Here's how the part is built. I have some questions about the finished solid (model axes, mm). Face numbers are marked on the shaded views. A direction names the side the tool comes from. Coordinates: 2 decimals unless noted, no trailing zeros. Write each loop counter-clockwise with the first axis right and the second up, starting at its lowest first coordinate (ties: lowest second). Pieces come first, ordered by that corner, then holes. Notation, with made-up numbers: M 25.25,88 L 59.25,88 A23 ccw 59.25,102 Z; hole C 29.5,41.5 d5. An arc over 180 degrees is marked long. Use one line per item in the form item = value. Start each with the question number.
1. Please list where these lines run through material, in increasing order: line 1 along Z through (x, y) = (30, -7.75); line 2 along X through (y, z) = (-1.25, -7); line 3 along Z through (x, y) = (28.5, -3.25). Write a range as [from, to].
2. I want a section at B-B, the plane y = -2.5. Count the separate pieces of the cut face and the enclosed holes in it, plus the area to 3 significant figures.
3. I'm going to push flat-ended pins straight in: pin 1 Ø5 at (x, y) = (33.5, -3) entering from +Z; pin 2 Ø11 at (y, z) = (-7, -0.5) entering from -X; pin 3 Ø1.5 at (x, z) = (-10.5, -3) entering from -Y. Where does each tip first touch, or does it pass through?
4. I want a section at C-C, the plane x = 3. List the corners of the cut face in (y, z) for me, plus the area to 3 significant figures.
5. I want a section at A-A, the plane z = 12. List the corners of the cut face in (x, y) for me, plus the area to 3 significant figures.
6. On a 3-axis mill with a long thin cutter (end or side, diameter ignored), from which of +Z, -Z, +X, -X, +Y, -Y can I reach the whole of each face in a straight line? I mean the marked faces 5, 6, 7, 8 and 9. Say none if no direction works.
7. Thinking about a two-plate mould opening in X: for the marked faces 1, 2, 3 and 4, which applies, released by +X, released by -X, zero draft, split by the parting line, or undercut?
from build123d import *
from build123d.topology import SkipClean

# Parameters (mm, degrees)
EXTRUDE_1_DEPTH       = 20
EXTRUDE_1_DEPTH_BACK  = 20
EXTRUDE_2_DEPTH       = 15
EXTRUDE_2_DEPTH_BACK  = 15
HOLE_WIZARD_M51_D     = 4.2
HOLE_WIZARD_M51_DEPTH = 16
HOLE_WIZARD_M51_TIP   = 1.2618073
CHAMFER_1_SIZE        = 3
FILLET_1_R            = 0.2
FILLET_2_R            = 0.2
FILLET_3_R            = 0.2


with BuildPart() as part:
    # Эскиз1 → Бобышка-Вытянуть1 (new, two sides: drawn at the far end of the back side and taken through both)
    with BuildSketch(Plane.XY.offset(-EXTRUDE_1_DEPTH_BACK)):
        with BuildLine():
            Line((17.5, -12.5), (7.5, -12.5))
            Line((7.5, -12.5), (7.5, -20))
            Line((7.5, -20), (-7.5, -20))
            Line((-7.5, -20), (-7.5, -12.5))
            Line((-7.5, -12.5), (-17.5, -12.5))
            ThreePointArc((-17.5, -12.5), (-26.338834765, -8.838834765), (-30, 0))
            Line((-30, 0), (-25, 0))
            ThreePointArc((-25, 0), (-17.5, -7.5), (-10, 0))
            Line((-10, 0), (10, 0))
            ThreePointArc((10, 0), (17.5, -7.5), (25, 0))
            Line((25, 0), (30, 0))
            ThreePointArc((30, 0), (26.338834765, -8.838834765), (17.5, -12.5))
        make_face()
    extrude(amount=EXTRUDE_1_DEPTH + EXTRUDE_1_DEPTH_BACK)

    # Эскиз2 → Бобышка-Вытянуть2 (add, two sides: drawn at the far end of the back side and taken through both)
    with SkipClean():  # the faces are left unmerged after this step: merging them gives an invalid solid
        with BuildSketch(Plane.XY.offset(-EXTRUDE_2_DEPTH_BACK)):
            with BuildLine():
                Line((22.5, -25), (45, -25))
                Line((45, -25), (45, -10))
                Line((45, -10), (35, -10))
                Line((35, -10), (35, 0))
                Line((35, 0), (25, 0))
                ThreePointArc((25, 0), (17.5, -7.5), (10, 0))
                Line((10, 0), (-10, 0))
                ThreePointArc((-10, 0), (-17.5, -7.5), (-25, 0))
                Line((-25, 0), (-35, 0))
                Line((-35, 0), (-35, -10))
                Line((-35, -10), (-45, -10))
                Line((-45, -10), (-45, -25))
                Line((-45, -25), (-22.5, -25))
                Line((-22.5, -25), (-27.5, -20))
                Line((-27.5, -20), (27.5, -20))
                Line((27.5, -20), (22.5, -25))
            make_face()
        extrude(amount=EXTRUDE_2_DEPTH + EXTRUDE_2_DEPTH_BACK)
    add(part.part.scale(1), mode=Mode.REPLACE)  # the faces are merged on a copy

    # Отверстие обработанное метчиком M51
    with Locations(Plane(origin=(0, 0, 0), x_dir=(1, 0, 0), z_dir=(0, 1, 0))):
        with Locations((-30, 7.5), (-30, -7.5), (0, 15), (0, -15), (30, -7.5), (30, 7.5)):
            Hole(HOLE_WIZARD_M51_D / 2, depth=HOLE_WIZARD_M51_DEPTH)
            with Locations((0, 0, -(HOLE_WIZARD_M51_DEPTH + HOLE_WIZARD_M51_TIP / 2))):  # 118° drill point
                Cone(0, HOLE_WIZARD_M51_D / 2, HOLE_WIZARD_M51_TIP, mode=Mode.SUBTRACT)

    # Фаска1
    chamfer_1_edges = [part.edges().sort_by_distance(p)[0] for p in [
        (-45, -10, 0),
        (45, -10, 0),
    ]]
    chamfer(chamfer_1_edges, length=CHAMFER_1_SIZE)

    # Скругление1
    fillet_1_edges = [part.edges().sort_by_distance(p)[0] for p in [
        (27.5, -20, 0),
        (22.5, -25, 0),
        (-27.5, -20, 0),
        (-22.5, -25, 0),
    ]]
    fillet(fillet_1_edges, radius=FILLET_1_R)

    # Скругление2
    fillet_2_edges = [part.edges().sort_by_distance(p)[0] for p in [
        (-35, -10, 0),
    ]]
    fillet(fillet_2_edges, radius=FILLET_2_R)

    # Скругление3
    fillet_3_edges = [part.edges().sort_by_distance(p)[0] for p in [
        (-12.5, -12.5, 15),
        (-12.5, -12.5, -15),
        (12.5, -12.5, -15),
        (26.338834765, -8.838834765, -15),
        (7.5, -16.25, -15),
        (12.5, -12.5, 15),
        (26.338834765, -8.838834765, 15),
        (-26.338834765, -8.838834765, 15),
        (-7.5, -16.25, 15),
        (7.5, -16.25, 15),
        (-26.338834765, -8.838834765, -15),
        (-7.5, -16.25, -15),
    ]]
    fillet(fillet_3_edges, radius=FILLET_3_R)


solid = part.part
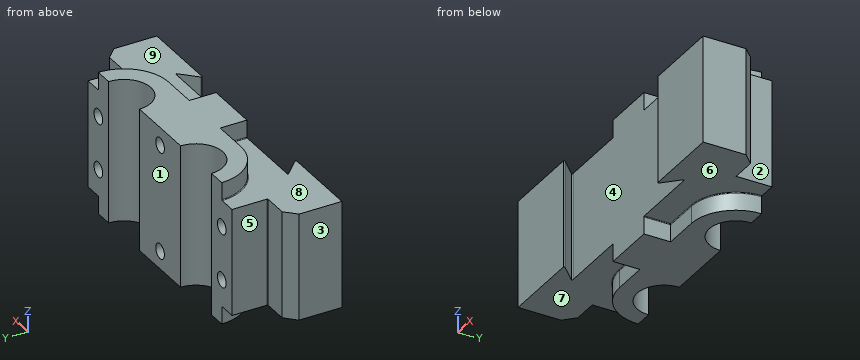
Answer list:
q1.line_1 = [-15, -9.6], [-5.4, 5.4], [9.6, 15]
q1.line_2 = [-35, -32.04], [-27.96, -24.9], [-10.1, 10.1], [24.9, 27.96], [32.04, 35]
q1.line_3 = [-20, -8.97], [-6.03, 6.03], [8.97, 20]
q2.separate_pieces = 3
q2.enclosed_holes = 6
q2.area = 1,480 mm²
q3.pin_1 = 15
q3.pin_2 = -44.5
q3.pin_3 = -20
q4.outline = M -20,-20 L 0,-20 L 0,20 L -20,20 Z
q4.area = 800 mm²
q5.outline = M -45,-25 L -22.98,-25 A0.2 ccw -22.84,-24.66 L -27.16,-20.34 A0.2 cw -27.02,-20 L 27.02,-20 A0.2 cw 27.16,-20.34 L 22.84,-24.66 A0.2 ccw 22.98,-25 L 45,-25 L 45,-13 L 42,-10 L 35,-10 L 35,0 L 25,0 A7.5 cw 10,0 L -10,0 A7.5 cw -25,0 L -35,0 L -35,-9.8 A0.2 cw -35.2,-10 L -42,-10 L -45,-13 Z
q5.area = 1,610 mm²
q6.face_5 = +Z, -Z, -X, +Y
q6.face_6 = -Z, +X, -Y
q6.face_7 = -Z, -X, -Y
q6.face_8 = +Z, -X, -Y
q6.face_9 = +Z, +X, -Y
q7.face_1 = zero draft
q7.face_2 = released by +X
q7.face_3 = released by -X
q7.face_4 = undercut
